Input: part model. Units: mm. Frame: model coordinates. A direction names the side the tool comes from. Round coordinates to 2 decimals unless told otherwise and drop trailing zeros. Loops run counter-clockwise (first coordinate to the right, second up) from the corner with the lowest first, then second, coordinate; pieces in that order, holes last. Notation, with made-up numbers: (-21.5, 55.5) -> (30.5, 55.5) arc R21 ccw to (30.5, 70.5) -> close; hole circle Ø8 at (41, 44.5). An arc over 180 degrees is marked (long way). Answer as a JSON object with one key per item and string values. Group by question number.
Item 1: Material intervals for line 1 (Y direction, x = 62.5, z = 22.5); line 2 (Y direction, x = 18, z = 3.5); line 3 (Z direction, x = 54.5, y = 2), sorted ascending. Write a range as [from, to].
Item 2: Set-up query: faces 1 (the flat face through (32.307, -16.567, 13.19)), 2 (the flat face through (32.307, -11.105, 11.607)). Return all of +Z, -Z, +X, -X, +Y, -Y with unobstructed straight access to the full face (end or side cutting, diameter ignored); none if empty.
Item 3: Section query B-B on y = -15. Return loops of the section in (x, z).
Item 4: Section query A-A on z = 15.5. Return loops of the section in (x, y).
Item 5: Pin query (flat end, axial travel): pin 1 (4 mm diameter, centred on x = 19, z = 18, fed in from -Y); pin 2 (6 mm diameter, centred on x = 15.5, y = 0.5, fed in from -Z); pin 3 (6 mm diameter, centred on x = 32.5, z = 35, fed in from -Y). Return the tip coordinate at first contact, or that it passes through.
from build123d import *

# Parameters (mm, degrees)
F1_DEPTH = 65.532
F3_DEPTH = 25.4


with BuildPart() as f1:
    # F0 (on Right) → F1 (new body)
    with BuildSketch(Plane.YZ):
        Polygon((9.926255, 54.951947), (-24.934381, 0), (-18.468346, 0), (14.536806, 52.027088), align=None)
    extrude(amount=F1_DEPTH)

    # F2 (on face) → F3 (cut)
    with BuildSketch(Plane(origin=(0, -17.779247, 11.27887), x_dir=(1, 0, 0), z_dir=(0, -0.844418, 0.535685))):
        Polygon((-17.95695, 38.16301), (0, 9.537645), (65.532, 26.100498), (82.354724, 60.764659), (0, 74.19014), align=None)
    extrude(amount=-F3_DEPTH, mode=Mode.SUBTRACT)

    # F5 (on face) → F6 section 0
    with BuildSketch(Plane(origin=(0, 0, 0), x_dir=(0, -1, 0), z_dir=(-1, 0, 0))):
        Polygon((-8.362336, 27.253337), (8.059522, 16.407767), (12.670072, 19.332627), (-5.352806, 31.810228), align=None)
    # F4 (on face) → F6 section 1
    with BuildSketch(Plane.YZ.offset(65.532)):
        Polygon((-3.797598, 33.318595), (0.812953, 30.393735), (16.414955, 39.848458), (13.584736, 44.518831), align=None)
    loft()


solid = f1.part
Solved:
{
 "1": {"line 1": "[-10.66, -4.19]", "line 2": "[-22.71, -16.25]", "line 3": "[29.69, 35.72]"},
 "2": {"face 1": "+Z, +X, -X, -Y", "face 2": "-Z, +X, +Y"},
 "3": {"outline": "(0, 5.47) -> (65.53, 5.47) -> (65.53, 15.66) -> (0, 15.66) -> close"},
 "4": {"outline": "(0, -15.1) -> (65.53, -15.1) -> (65.53, -8.64) -> (0, -8.64) -> close"},
 "5": {"pin 1": "y = -14.78", "pin 2": "z = 21.92", "pin 3": "y = 0.27"}
}
